The listing builds one solid part. Answer for the finished solid, in the listing's coordinates (mm). A direction names the side the tool comes from. Coordinates: 2 decimals unless noted, no trailing zeros. Loops run counter-clockwise (first coordinate to the right, second up) from the corner with the lowest first, then second, coordinate; pieces in that order, holes last. Notation, with made-up numbers: M 84,-23 L 89,-23 A9 cw 89,-12 Z; hole C -3.5,35 d4. An arc over 180 degrees is marked long. Answer as CSV lines item,"result". Start each with the question number.
```python
from build123d import *

# Parameters (mm, degrees)
BOSS_EXTRUDE1_START = 11.1125
BOSS_EXTRUDE1_DEPTH = 22.225
FILLET1_R           = 1.2715875
SKETCH4_R           = 3.5687
CUT_EXTRUDE1_DEPTH  = 54.741037043
SKETCH6_R           = 3.5687
CUT_EXTRUDE3_DEPTH  = 7.874
CHAMFER1_SIZE       = 0.508
FILLET2_R           = 0.254


with BuildPart() as part:
    # Sketch3 → Boss-Extrude1 (new body)
    with BuildSketch(Plane(origin=(0, 0, 0), x_dir=(0, 0, -1), z_dir=(1, 0, 0)).offset(BOSS_EXTRUDE1_START)):
        with BuildLine():
            Line((-3.175, -20.6375), (-41.275, -20.6375))
            ThreePointArc((-41.275, -20.6375), (-44.642596045, -22.032403955), (-46.0375, -25.4))
            Line((-46.0375, -25.4), (4.7625, -25.4))
            Line((4.7625, -25.4), (4.7625, 25.4))
            ThreePointArc((4.7625, 25.4), (1.394903955, 24.005096045), (0, 20.6375))
            Line((0, 20.6375), (0, -17.4625))
            ThreePointArc((0, -17.4625), (-0.92993597, -19.70756403), (-3.175, -20.6375))
        make_face()
    extrude(amount=-BOSS_EXTRUDE1_DEPTH)

    # Fillet1
    fillet1_edges = [part.edges().sort_by_distance(p)[0] for p in [
        (0, -25.4, -4.7625),
    ]]
    fillet(fillet1_edges, radius=FILLET1_R)

    # Sketch4 → Cut-Extrude1 (cut, through all)
    with BuildSketch(Plane.XY):
        with Locations((0, 12.7)):
            Circle(SKETCH4_R)
        with Locations(Location((0, -12.7, 0), (0, 0, 180))):
            Circle(SKETCH4_R)
    extrude(amount=-CUT_EXTRUDE1_DEPTH, mode=Mode.SUBTRACT)

    # Sketch6 → Cut-Extrude3 (cut)
    with BuildSketch(Plane(origin=(0, -20.6375, 0), x_dir=(1, 0, 0), z_dir=(0, 1, 0))):
        with Locations(Location((0, -7.9375, 0), (0, 0, 270))):
            Circle(SKETCH6_R)
        with Locations(Location((0, -33.3375, 0), (0, 0, 270))):
            Circle(SKETCH6_R)
    extrude(amount=-CUT_EXTRUDE3_DEPTH, mode=Mode.SUBTRACT)

    # Chamfer1
    chamfer1_edges = [part.edges().sort_by_distance(p)[0] for p in [
        (-3.5687, 12.7, 0),
        (3.5687, -12.7, 0),
        (0, -20.6375, 4.3688),
        (0, -20.6375, 29.7688),
    ]]
    chamfer(chamfer1_edges, length=CHAMFER1_SIZE)

    # Fillet2
    fillet2_edges = [part.edges().sort_by_distance(p)[0] for p in [
        (0, 25.4, -4.7625),
        (-11.1125, 24.005096045, -1.394903955),
        (-11.1125, 1.5875, 0),
        (-11.1125, -19.70756403, 0.92993597),
        (-11.1125, -20.6375, 22.225),
        (11.1125, 0.63579375, -4.7625),
        (11.1125, -25.027560644, -4.390060644),
        (-11.1125, 0.63579375, -4.7625),
        (-11.1125, -25.027560644, -4.390060644),
        (-3.5687, 12.7, -4.7625),
        (3.5687, -12.7, -4.7625),
        (-11.1125, -22.032403955, 44.642596045),
        (11.1125, -20.6375, 22.225),
        (-11.1125, -25.4, 21.27329375),
        (11.1125, -19.70756403, 0.92993597),
        (11.1125, 1.5875, 0),
        (11.1125, 24.005096045, -1.394903955),
        (11.1125, -25.4, 21.27329375),
        (11.1125, -22.032403955, 44.642596045),
    ]]
    fillet(fillet2_edges, radius=FILLET2_R)


solid = part.part
```
Item 1: For a pull along Z with two mould halves and no side action, classify faces 3 (the face through (-11.112, -22, 10)), 4 (the face through (1.07, -23.24, 11.34)), 5 (the face through (0.15, 23.95, -1.34)) as pulls with the +Z half, pulls with the -Z half, needs draft (parallel to the pull), parting line crosses it, or undercut.
Item 2: For faces 1 (the face through (0, -20.638, 22)), 2 (the face through (-0.15, -25.04, -4.38)), determine the directions among +Z, -Z, +X, -X, +Y, -Y from which every point of the face is accessible in a straight line to the end or side of a thin tool.
Item 3: Section B-B on y = 5 is taken. Determine the outline of the cut face in (x, z), then the cut area to 3 significant figures.
Item 4: Consider line 1 (Y direction, x = 9.75, z = 34); line 2 (Z direction, x = -3.5, y = 4.5); line 3 (Y direction, x = 0, z = -2.85). Determine where each line is inside the solid, lowest interval first.
Item 5: Section A-A on y = -12.7 is taken. Determine the outline of the cut face in (x, z).
Item 6: Section D-D on z = 14 is taken. Determine the outline of the cut face in (x, y).
Item 7: Each of these flat-tipped pins is pushed along its axis until it touches: P1, Ø9.5, axis at x = 0, y = 12.7, coming from the -Z side; P2, Ø12, axis at x = -7, y = 8, coming from the +Z side; P3, Ø6.5, axis at x = 0, z = 33.34, coming from the +Y side; P4, Ø11, axis at x = -4, z = 25, coming from the +Y side. Where does it stop, or does it pass through?
Results are:
1,face 3,"needs draft"
1,face 4,"undercut"
1,face 5,"pulls with the +Z half"
2,face 1,"+Z, +X, -X, +Y"
2,face 2,"-Z, +X, -X, -Y"
3,outline,"M -11.11,-4.51 A0.25 ccw -10.86,-4.76 L 10.86,-4.76 A0.25 ccw 11.11,-4.51 L 11.11,-0.25 A0.25 ccw 10.86,0 L -10.86,0 A0.25 ccw -11.11,-0.25 Z"
3,area,"106 mm²"
4,line 1,"-25.4 to -20.64"
4,line 2,"-4.76 to 0"
4,line 3,"-25.4 to -16.27, -9.13 to 9.13, 16.27 to 25"
5,outline,"M -11.11,-4.51 A0.25 ccw -10.86,-4.76 L -3.82,-4.76 A0.25 ccw -3.57,-4.51 L -3.57,-0.51 L -4.08,0 L -10.86,0 A0.25 ccw -11.11,-0.25 Z; M 3.57,-4.51 A0.25 ccw 3.82,-4.76 L 10.86,-4.76 A0.25 ccw 11.11,-4.51 L 11.11,-0.25 A0.25 ccw 10.86,0 L 4.08,0 L 3.57,-0.51 Z"
6,outline,"M -11.11,-25.15 A0.25 ccw -10.86,-25.4 L 10.86,-25.4 A0.25 ccw 11.11,-25.15 L 11.11,-20.89 A0.25 ccw 10.86,-20.64 L -10.86,-20.64 A0.25 ccw -11.11,-20.89 Z"
7,P1,"z = -4.76"
7,P2,"z = 0"
7,P3,"through"
7,P4,"y = -20.64"
